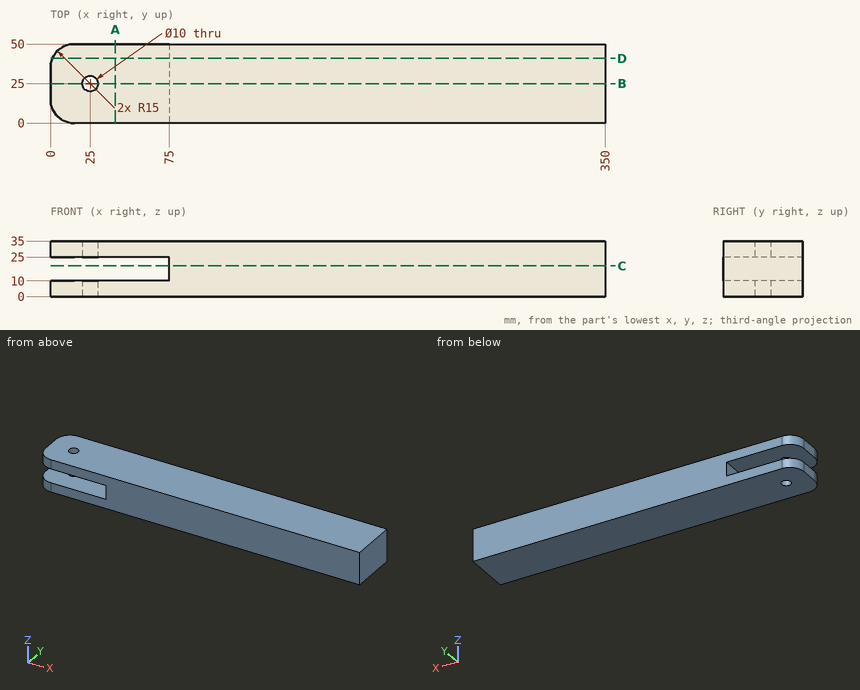
Could you check a few things on this drawing? It's one solid part, dimensions in mm from its lowest x, y, z. Coordinates: 2 decimals unless noted, no trailing zeros. Order: outer loops, then holes, each group sorted by start corner. A loop starts at its lowest first (then second) coordinate and runs counter-clockwise, first axis right, second up. Notation, with made-up numbers: M 5.25,-33 L 53.25,-33 A11 ccw 53.25,-14 Z; hole C 8.25,18 d1. An arc over 180 degrees is marked long. Use one line per item in the form item = value. Start each with the question number.
1. Suppose I cut it at A-A on x = 41. Write out the boundary of the cut face in (y, z), then the cut area to 3 significant figures.
2. Suppose I cut it at D-D on y = 41. Write out the boundary of the cut face in (x, z).
3. For pin 1 (8 mm diameter, centred on x = 302.5, z = 21, fed in from -Y); pin 2 (6 mm diameter, centred on x = 25, y = 25, fed in from +Z); pin 3 (4.5 mm diameter, centred on y = 34.5, z = 18.5, fed in from -X), each with a flat end and sliding along its axis, tell me the tip position at first contact or that it passes through.
4. Suppose I cut it at B-B on y = 25. Write out the boundary of the cut face in (x, z).
5. Suppose I cut it at C-C on z = 19.5. Write out the boundary of the cut face in (x, y).
6. Please list where these lines run through material, in increasing order: line 1 (Z direction, x = 46, y = 24.5); line 2 (X direction, y = 25, z = 5); line 3 (Y direction, x = 25, z = 31).
Geometry says:
q1.outline = M 0,0 L 50,0 L 50,10 L 0,10 Z; M 0,25 L 50,25 L 50,35 L 0,35 Z
q1.area = 1,000 mm^2
q2.outline = M 1.25,0 L 350,0 L 350,35 L 1.25,35 L 1.25,25 L 75,25 L 75,10 L 1.25,10 Z
q3.pin_1 = 0
q3.pin_2 = through
q3.pin_3 = 75
q4.outline = M 0,0 L 20,0 L 20,10 L 0,10 Z; M 0,25 L 20,25 L 20,35 L 0,35 Z; M 30,0 L 350,0 L 350,35 L 30,35 L 30,25 L 75,25 L 75,10 L 30,10 Z
q5.outline = M 75,0 L 350,0 L 350,50 L 75,50 Z
q6.line_1 = 0 to 10, 25 to 35
q6.line_2 = 0 to 20, 30 to 350
q6.line_3 = 0 to 20, 30 to 50
